from build123d import *

# Parameters (mm, degrees)
F0_W          = 70
F0_H          = 70
F1_DEPTH      = 10
F2_T          = -2
F3_W          = 66
F3_H          = 8
F4_DEPTH      = 4.32812
F5_R          = 0.5
F6_DEPTH      = 2.001
F6_DEPTH_BACK = 68.001


with BuildPart() as f1:
    # F0 (on Front) → F1 (new body)
    with BuildSketch(Plane.XZ):
        with Locations((0, -7.2107579758)):
            Rectangle(F0_W, F0_H)
    extrude(amount=F1_DEPTH)

    # F2
    f2_openings = [f1.faces().sort_by_distance(p)[0] for p in [
        (0, 0, -7.210758),
    ]]
    offset(amount=F2_T, openings=f2_openings)

    # F3 (on face) → F4 (cut)
    with BuildSketch(Plane.XY.offset(27.7892420242)):
        with Locations((0, -4)):
            Rectangle(F3_W, F3_H)
    extrude(amount=-F4_DEPTH, mode=Mode.SUBTRACT)

    # F5 (on face) → F6 (cut, two sides)
    with BuildSketch(Plane(origin=(33, 0, 0), x_dir=(0, -1, 0), z_dir=(-1, 0, 0))) as f6_sk:
        with Locations((4, 22.7892420242)):
            Circle(F5_R)
        with Locations((4, -35.2107579758)):
            Circle(F5_R)
    extrude(amount=-F6_DEPTH, mode=Mode.SUBTRACT)
    extrude(f6_sk.sketch, amount=F6_DEPTH_BACK, mode=Mode.SUBTRACT)


solid = f1.part
Source: CAD feature listing. Evaluate the final solid. Frame: model axes, mm. A direction names the side the tool comes from. Give positions to 0.01 mm unless a question says otherwise; leave off trailing zeros. Loops run counter-clockwise (first coordinate to the right, second up) from the corner with the lowest first, then second, coordinate; pieces in that order, holes last. Notation, with made-up numbers: (-15.5, 58.5) -> (35.5, 58.5) arc R22 cw to (35.5, 77.5) -> close; hole circle Ø3 at (-34.75, -32.75). An arc over 180 degrees is marked (long way). Use a Markdown table: item, result. Add a question column.
1) Section query C-C, the plane z = 14.5. Return the cut outline in (x, y), then the cut area to 3 significant figures.
2) First-contact query: pin 1 (1.5 mm diameter, centred on x = -12.5, z = -24.5, fed in from +Y); pin 2 (4 mm diameter, centred on x = 9, y = -2.5, fed in from +Z). Flat tips, straight axial feed; report the tip coordinate or a pass-through.
3) Section query B-B, the plane x = -10. Return the cut outline in (y, z), then the cut area to 3 significant figures.
4) Line query: line 1 along Z through (x, y) = (-33.85, -4); line 2 along X through (y, z) = (-1.75, -30); line 3 along Y through (x, z) = (20, 10). Output: solid intervals per line, ascending. Write a range as [from, to].
5) Section query A-A, the plane y = -6.5. Return the cut outline in (x, z).
6) Pull-direction query (X, two-part tool) for faces 1 (the face through (0, 0, -41)), 2 (the face through (-35, -5, -8)), 3 (the face through (-33, -4, -6)), 4 (the face through (33, -4, -6)); classes: +X half, -X half, draft (parallel to the pull), parting line (faces both ways), or undercut.
7) Reachability of faces 5 (the face through (0, -5, -42.211)), 6 (the face through (0, -4, -40.211)) from +Z, -Z, +X, -X, +Y, -Y: full face, straight path, thin tool, end or side. Return the list, or none.
Numbers:
| question | item | result |
|---|---|---|
| 1 | outline | (-35, -10) -> (35, -10) -> (35, 0) -> (33, 0) -> (33, -8) -> (-33, -8) -> (-33, 0) -> (-35, 0) -> close |
| 1 | area | 172 mm2 |
| 2 | pin 1 | stops at y = -8 |
| 2 | pin 2 | stops at z = -40.21 |
| 3 | outline | (-10, -42.21) -> (0, -42.21) -> (0, -40.21) -> (-8, -40.21) -> (-8, 27.79) -> (-10, 27.79) -> close |
| 3 | area | 156 mm2 |
| 4 | line 1 | z = [-42.21, -35.71], [-34.71, 22.29], [23.29, 27.79] |
| 4 | line 2 | x = [-35, -33], [33, 35] |
| 4 | line 3 | y = [-10, -8] |
| 5 | outline | (-35, -42.21) -> (35, -42.21) -> (35, 27.79) -> (33, 27.79) -> (33, -40.21) -> (-33, -40.21) -> (-33, 27.79) -> (-35, 27.79) -> close |
| 6 | face 1 | draft |
| 6 | face 2 | -X half |
| 6 | face 3 | undercut |
| 6 | face 4 | undercut |
| 7 | face 5 | -Z, +X, -X, +Y, -Y |
| 7 | face 6 | +Z, +Y |
